```python
from build123d import *

# Parameters (mm, degrees)
AUFSATZ_LINEAR_AUSTRAGEN2_DEPTH = 5
AUFSATZ_LINEAR_AUSTRAGEN3_DEPTH = 30
FASE3_SIZE                      = 25
SKIZZE3_R                       = 1.6
SCHNITT_LINEAR_AUSTRAGEN2_DEPTH = 30
SKIZZE4_R                       = 1.6
SCHNITT_LINEAR_AUSTRAGEN3_DEPTH = 30
SKIZZE5_R                       = 1.6
SCHNITT_LINEAR_AUSTRAGEN4_DEPTH = 30


with BuildPart() as part:
    # Skizze1 → Aufsatz-Linear austragen2 (new body)
    with BuildSketch(Plane.XY):
        Polygon((5, 30), (5, 5), (30, 5), align=None)
    extrude(amount=AUFSATZ_LINEAR_AUSTRAGEN2_DEPTH)

    # Skizze1_5 → Aufsatz-Linear austragen3 (add)
    with BuildSketch(Plane.XY):
        Polygon((5, 5), (30, 5), (30, 0), (0, 0), (0, 30), (5, 30), align=None)
    extrude(amount=AUFSATZ_LINEAR_AUSTRAGEN3_DEPTH)

    # Fase3
    fase3_edges = [part.edges().sort_by_distance(p)[0] for p in [
        (2.5, 30, 30),
        (30, 2.5, 30),
    ]]
    chamfer(fase3_edges, length=FASE3_SIZE)

    # Skizze3 → Schnitt-Linear austragen2 (cut)
    with BuildSketch(Plane(origin=(0, 5, 0), x_dir=(1, 0, 0), z_dir=(0, 1, 0))):
        with Locations(Location((15, -15, 0), (0, 0, 270))):
            Circle(SKIZZE3_R)
    extrude(amount=-SCHNITT_LINEAR_AUSTRAGEN2_DEPTH, mode=Mode.SUBTRACT)

    # Skizze4 → Schnitt-Linear austragen3 (cut)
    with BuildSketch(Plane(origin=(5, 0, 0), x_dir=(0, 0, -1), z_dir=(1, 0, 0))):
        with Locations(Location((-15, 15, 0), (0, 0, 90))):
            Circle(SKIZZE4_R)
    extrude(amount=-SCHNITT_LINEAR_AUSTRAGEN3_DEPTH, mode=Mode.SUBTRACT)

    # Skizze5 → Schnitt-Linear austragen4 (cut)
    with BuildSketch(Plane.XY.offset(5)):
        with Locations((15, 15)):
            Circle(SKIZZE5_R)
    extrude(amount=-SCHNITT_LINEAR_AUSTRAGEN4_DEPTH, mode=Mode.SUBTRACT)


solid = part.part
```
CAD build for the part. Positions are in the model's coordinates, mm. A direction names the side the tool comes from. Round coordinates to 2 decimals unless told otherwise and drop trailing zeros. Write each loop counter-clockwise with the first axis right and the second up, starting at its lowest first coordinate (ties: lowest second). Pieces come first, ordered by that corner, then holes. Notation, with made-up numbers: M 61.25,16.5 L 82.25,16.5 A29 ccw 82.25,50.5 Z; hole C 28,-18.5 d9. An arc over 180 degrees is marked long. One line per question, with ' | ' between items.
1. Which spindle directions (+Z, -Z, +X, -X, +Y, -Y) get a long thin tool onto all of the face, cutting with end or side? Do faces 5 (the flat face through (12, 12, 5)), 6 (the flat face through (2, 30, 2)). Say none if no direction does.
Working result:
face 5: +Z, +X, +Y | face 6: +Z, -Z, +X, -X, +Y
2. Cut at D-D on y = 28. Write the cut outline in (x, z), and give its area (3 significant figures).
Working result:
outline: M 0,0 L 7,0 L 7,5 L 5,5 L 5,7 L 0,7 Z | area: 45.0 mm2
3. Cut at C-C on z = 3.5. Write the cut outline in (x, y), and give its area (3 significant figures).
Working result:
outline: M 0,0 L 30,0 L 30,5 L 5,30 L 0,30 Z; hole C 15,15 d3.2 | area: 579 mm2
4. Probe L1, parallel to Z at x = 19.25, y = 10. List the from-to ranges inside material, lowest first. Write a range as from..to.
Working result:
L1: 0..5
5. Pin check, flat tips, straight feed: pin 1 Ø4 at (y, z) = (15, 15) entering from +X; pin 2 Ø5 at (x, y) = (15, 15) entering from +Z; pin 3 Ø5 at (x, y) = (5.5, 9.5) entering from +Z; pin 4 Ø12.5 at (x, z) = (21, 23.5) entering from +Y. Stop position of each tip, or through.
Working result:
pin 1: x = 5 | pin 2: z = 5 | pin 3: z = 27.95 | pin 4: through
6. Mould opens along Y. For faces 1 (the cylindrical face through (2.54, 13.4, 15.07)), 2 (the flat face through (2, 18, 17)), 3 (the cylindrical face through (13.4, 15.07, 2.54)), 4 (the flat face through (3, 3, 30)) say: pulls with the +Y half, pulls with the -Y half, needs draft (parallel to the pull), parting line crosses it, or undercut.
Working result:
face 1: undercut | face 2: pulls with the +Y half | face 3: undercut | face 4: needs draft
7. Cut at A-A on y = 15. Write the cut outline in (x, z).
Working result:
outline: M 0,0 L 13.4,0 L 13.4,5 L 5,5 L 5,13.4 L 0,13.4 Z; M 0,16.6 L 5,16.6 L 5,20 L 0,20 Z; M 16.6,0 L 20,0 L 20,5 L 16.6,5 Z
